```python
from build123d import *

# Parameters (mm, degrees)
SKETCH1_R                           = 25.4
BOSS_EXTRUDE1_DEPTH                 = 25.4
SKETCH2_R                           = 16
CUT_EXTRUDE1_DEPTH                  = 21.59
CUT_EXTRUDE2_REACH                  = 45.994
CUT_EXTRUDE2_END_RADIUS             = 25.4
SKETCH3_W                           = 3.175
SKETCH3_H                           = 16.51
CUT_EXTRUDE2_DIRECTION_2_REACH      = 45.994
CUT_EXTRUDE2_DIRECTION_2_END_RADIUS = 25.4
CUT_EXTRUDE3_REACH                  = 43.91
SKETCH4_R                           = 1
CUT_EXTRUDE4_REACH                  = 41.534


with BuildPart() as part:
    # Sketch1 → Boss-Extrude1 (new body)
    with BuildSketch(Plane(origin=(0, 0, 0), x_dir=(1, 0, 0), z_dir=(0, 1, 0))):
        with Locations(Location((0, 0, 0), (0, 0, 270))):
            Circle(SKETCH1_R)
    extrude(amount=BOSS_EXTRUDE1_DEPTH)

    # Sketch2 → Cut-Extrude1 (cut)
    with BuildSketch(Plane(origin=(0, 25.4, 0), x_dir=(1, 0, 0), z_dir=(0, 1, 0))):
        with Locations(Location((0, 0, 0), (0, 0, 270))):
            Circle(SKETCH2_R)
    extrude(amount=-CUT_EXTRUDE1_DEPTH, mode=Mode.SUBTRACT)

    # Cut-Extrude2: up to this cylinder (the profile starts inside it)
    cut_extrude2_end = Plane(origin=(0, 17.145, 0), z_dir=(0, -1, 0)) * Cylinder(CUT_EXTRUDE2_END_RADIUS, 143.788, mode=Mode.PRIVATE)
    # Sketch3 → Cut-Extrude2 (cut, up to the surface)
    with BuildSketch(Plane.XY, mode=Mode.PRIVATE) as cut_extrude2_sk1:
        with Locations((23.8125, 17.145)):
            Rectangle(SKETCH3_W, SKETCH3_H)
    cut_extrude2_tool1 = extrude(cut_extrude2_sk1.sketch, amount=-CUT_EXTRUDE2_REACH, mode=Mode.PRIVATE) & cut_extrude2_end
    add(cut_extrude2_tool1.solids().sort_by_distance((23.8125, 17.145, 0))[0], mode=Mode.SUBTRACT)
    # Sketch3 → Cut-Extrude2 (cut, up to the surface)
    with BuildSketch(Plane.XY, mode=Mode.PRIVATE) as cut_extrude2_sk2:
        with Locations((-23.8125, 17.145)):
            Rectangle(SKETCH3_W, SKETCH3_H)
    cut_extrude2_tool2 = extrude(cut_extrude2_sk2.sketch, amount=-CUT_EXTRUDE2_REACH, mode=Mode.PRIVATE) & cut_extrude2_end
    add(cut_extrude2_tool2.solids().sort_by_distance((-23.8125, 17.145, 0))[0], mode=Mode.SUBTRACT)

    # Cut-Extrude2 direction 2: up to this cylinder (the profile starts inside it)
    cut_extrude2_direction_2_end = Plane(origin=(0, 17.145, 0), z_dir=(0, -1, 0)) * Cylinder(CUT_EXTRUDE2_DIRECTION_2_END_RADIUS, 143.788, mode=Mode.PRIVATE)
    # Sketch3 → Cut-Extrude2 direction 2 (cut, up to the surface)
    with BuildSketch(Plane.XY, mode=Mode.PRIVATE) as cut_extrude2_direction_2_sk1:
        with Locations((23.8125, 17.145)):
            Rectangle(SKETCH3_W, SKETCH3_H)
    cut_extrude2_direction_2_tool1 = extrude(cut_extrude2_direction_2_sk1.sketch, amount=CUT_EXTRUDE2_DIRECTION_2_REACH, mode=Mode.PRIVATE) & cut_extrude2_direction_2_end
    add(cut_extrude2_direction_2_tool1.solids().sort_by_distance((23.8125, 17.145, 0))[0], mode=Mode.SUBTRACT)
    # Sketch3 → Cut-Extrude2 direction 2 (cut, up to the surface)
    with BuildSketch(Plane.XY, mode=Mode.PRIVATE) as cut_extrude2_direction_2_sk2:
        with Locations((-23.8125, 17.145)):
            Rectangle(SKETCH3_W, SKETCH3_H)
    cut_extrude2_direction_2_tool2 = extrude(cut_extrude2_direction_2_sk2.sketch, amount=CUT_EXTRUDE2_DIRECTION_2_REACH, mode=Mode.PRIVATE) & cut_extrude2_direction_2_end
    add(cut_extrude2_direction_2_tool2.solids().sort_by_distance((-23.8125, 17.145, 0))[0], mode=Mode.SUBTRACT)

    # Sketch4 → Cut-Extrude3 (cut, up to next)
    with BuildSketch(Plane(origin=(0, 3.81, 0), x_dir=(1, 0, 0), z_dir=(0, 1, 0)), mode=Mode.PRIVATE) as cut_extrude3_sk1:
        with Locations(Location((0, 8.89, 0), (0, 0, 270))):
            Circle(SKETCH4_R)
    cut_extrude3_tool1 = extrude(cut_extrude3_sk1.sketch, amount=-CUT_EXTRUDE3_REACH, mode=Mode.PRIVATE) & part.part
    # Sketch4 → Cut-Extrude3 (cut, up to next)
    with BuildSketch(Plane(origin=(0, 3.81, 0), x_dir=(1, 0, 0), z_dir=(0, 1, 0)), mode=Mode.PRIVATE) as cut_extrude3_sk2:
        with Locations(Location((7.69896584, -4.445, 0), (0, 0, 270))):
            Circle(SKETCH4_R)
    cut_extrude3_tool2 = extrude(cut_extrude3_sk2.sketch, amount=-CUT_EXTRUDE3_REACH, mode=Mode.PRIVATE) & part.part
    # Sketch4 → Cut-Extrude3 (cut, up to next)
    with BuildSketch(Plane(origin=(0, 3.81, 0), x_dir=(1, 0, 0), z_dir=(0, 1, 0)), mode=Mode.PRIVATE) as cut_extrude3_sk3:
        with Locations(Location((-7.69896584, -4.445, 0), (0, 0, 270))):
            Circle(SKETCH4_R)
    cut_extrude3_tool3 = extrude(cut_extrude3_sk3.sketch, amount=-CUT_EXTRUDE3_REACH, mode=Mode.PRIVATE) & part.part
    add(cut_extrude3_tool1.solids().sort_by_distance((0, 3.81, -8.89))[0], mode=Mode.SUBTRACT)
    add(cut_extrude3_tool2.solids().sort_by_distance((7.698966, 3.81, 4.445))[0], mode=Mode.SUBTRACT)
    add(cut_extrude3_tool3.solids().sort_by_distance((-7.698966, 3.81, 4.445))[0], mode=Mode.SUBTRACT)

    # Sketch5 → Cut-Extrude4 (cut, up to next)
    with BuildSketch(Plane(origin=(0, 8.89, 0), x_dir=(1, 0, 0), z_dir=(0, 1, 0)), mode=Mode.PRIVATE) as cut_extrude4_sk1:
        with BuildLine():
            Line((22.225, 12.296722124), (22.225, -12.296722124))
            ThreePointArc((22.225, -12.296722124), (25.4, 0), (22.225, 12.296722124))
        make_face()
    cut_extrude4_tool1 = extrude(cut_extrude4_sk1.sketch, amount=-CUT_EXTRUDE4_REACH, mode=Mode.PRIVATE) & part.part
    # Sketch5 → Cut-Extrude4 (cut, up to next)
    with BuildSketch(Plane(origin=(0, 8.89, 0), x_dir=(1, 0, 0), z_dir=(0, 1, 0)), mode=Mode.PRIVATE) as cut_extrude4_sk2:
        with BuildLine():
            Line((-22.225, -12.296722124), (-22.225, 12.296722124))
            ThreePointArc((-22.225, 12.296722124), (-25.4, 0), (-22.225, -12.296722124))
        make_face()
    cut_extrude4_tool2 = extrude(cut_extrude4_sk2.sketch, amount=-CUT_EXTRUDE4_REACH, mode=Mode.PRIVATE) & part.part
    add(cut_extrude4_tool1.solids().sort_by_distance((23.502059, 8.89, 0))[0], mode=Mode.SUBTRACT)
    add(cut_extrude4_tool2.solids().sort_by_distance((-23.502059, 8.89, 0))[0], mode=Mode.SUBTRACT)


solid = part.part
```
Work out the finished part from the listing and answer in its coordinate system (mm). A direction names the side the tool comes from. Coordinates: 2 decimals unless noted, no trailing zeros. Order: outer loops, then holes, each group sorted by start corner. A loop starts at its lowest first (then second) coordinate and runs counter-clockwise, first axis right, second up. Notation, with made-up numbers: (30, 49) - (78, 49) arc R21 ccw to (78, 60) - close; hole circle Ø2 at (71.5, 78). An arc over 180 degrees is marked (long way). Answer as a JSON object with one key per item and string values.
1. Consider line 1 (X direction, y = 11.25, z = 0) (3 decimals); line 2 (X direction, y = 1.9, z = -8.89) (3 decimals); line 3 (Y direction, x = 9, z = 7.5). Determine where each line is inside the solid, lowest interval first.
Output values:
{"line 1": "x = -22.225 to -16, 16 to 22.225", "line 2": "x = -22.225 to -1, 1 to 22.225", "line 3": "y = 0 to 3.81"}
2. A tool of negligible diameter and unlimited length cuts with its end or side. For faces 1 (the face through (8.69, 1.93, 4.31)), 2 (the face through (0, 3.81, 0)), from which of +Z, -Z, +X, -X, +Y, -Y can it reach the whole face along a straight path? Write none if from no direction.
Output values:
{"face 1": "+Y, -Y", "face 2": "+Y"}
3. Find section D-D on z = 0. Determine the outline of the cut face in (x, y) (3 decimals).
Output values:
{"outline": "(-22.225, 0) - (22.225, 0) - (22.225, 25.4) - (16, 25.4) - (16, 3.81) - (-16, 3.81) - (-16, 25.4) - (-22.225, 25.4) - close"}
4. Find section A-A on x = 0. Determine the outline of the cut face in (y, z).
Output values:
{"outline": "(0, -25.4) - (25.4, -25.4) - (25.4, -16) - (3.81, -16) - (3.81, -9.89) - (0, -9.89) - close; (0, -7.89) - (3.81, -7.89) - (3.81, 16) - (25.4, 16) - (25.4, 25.4) - (0, 25.4) - close"}
5. The mould has two halves that part along Z. Classify faces 3 (the face through (-22.225, 13, 0)), 4 (the face through (0.379, 12.522, -25.397)), 5 (the face through (-0.379, 12.522, 25.397)), 6 (the face through (-15.62, 14.76, -3.47)): +Z half, -Z half, draft (parallel to the pull), parting line (faces both ways), or undercut.
Output values:
{"face 3": "draft", "face 4": "-Z half", "face 5": "+Z half", "face 6": "undercut"}
6. Find section C-C on y = 14.5. Determine the outline of the cut face in (x, z) (3 decimals), plus the area to 3 significant figures.
Output values:
{"outline": "(-22.225, -12.297) arc R25.4 ccw to (22.225, -12.297) - (22.225, 12.297) arc R25.4 ccw to (-22.225, 12.297) - close; hole circle Ø32 at (0, 0)", "area": "1,120 mm²"}
7. Each of these flat-tipped pins is pushed along its axis until it touches: P1, Ø9.5, axis at x = 7, z = -3.5, coming from the +Y side; P2, Ø6, axis at x = 11.5, z = 20, coming from the -Y side; P3, Ø3, axis at x = 9.5, y = 8.5, coming from the +Z side; P4, Ø4, axis at x = -14, y = 17, coming from the -Z side. Where does it stop, or does it pass through?
Output values:
{"P1": "stops at y = 3.81", "P2": "stops at y = 0", "P3": "stops at z = 24.11", "P4": "stops at z = -22.39"}
8. Find section B-B on z = -8.89. Determine the outline of the cut face in (x, y) (3 decimals), plus the area to 3 significant figures.
Output values:
{"outline": "(-22.225, 0) - (-1, 0) - (-1, 3.81) - (-13.303, 3.81) - (-13.303, 25.4) - (-22.225, 25.4) - close; (1, 0) - (22.225, 0) - (22.225, 25.4) - (13.303, 25.4) - (13.303, 3.81) - (1, 3.81) - close", "area": "547 mm²"}
